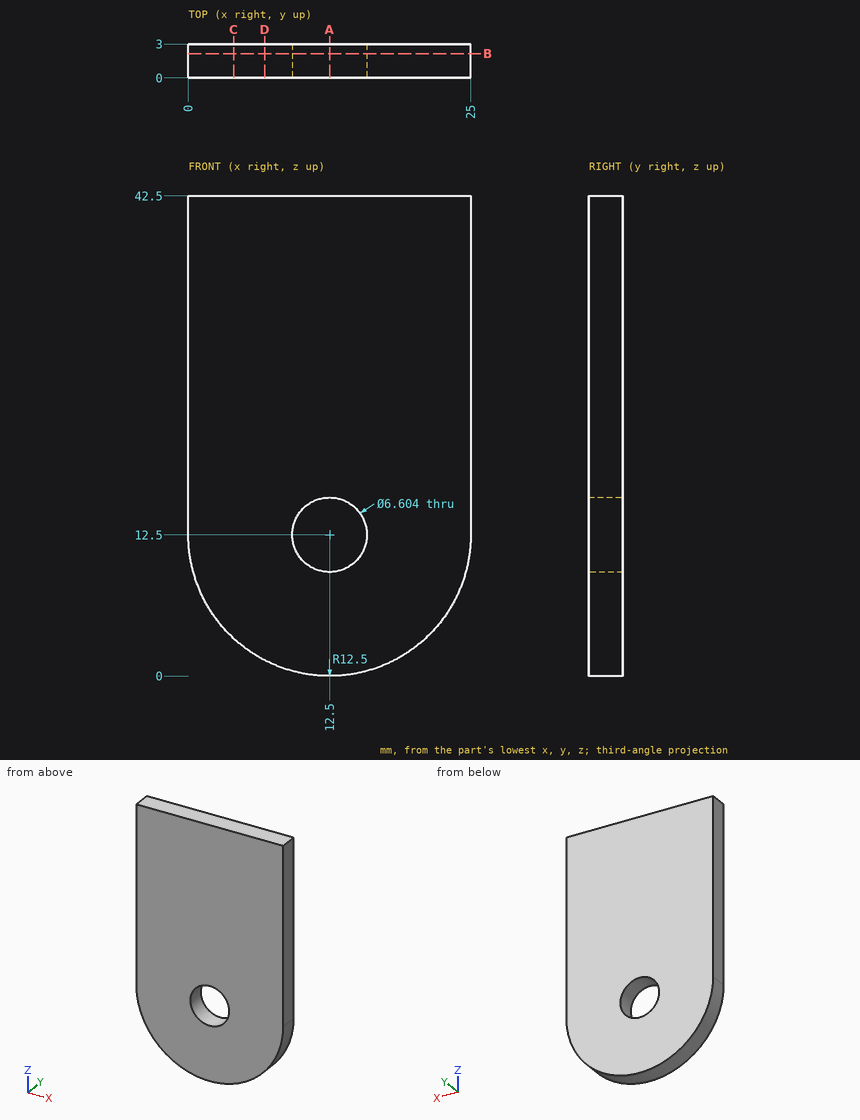
Job drawing, mm, ordinate dimensions from the low corner. One solid piece. Coordinates: 2 decimals unless noted, no trailing zeros. Write each loop counter-clockwise with the first axis right and the second up, starting at its lowest first coordinate (ties: lowest second). Pieces come first, ordered by that corner, then holes.
Item 1: Slice it at C-C (x = 4). Write the cut outline in (y, z), and give its area (3 significant figures).
Item 2: Slice it at B-B (y = 2.15). Write the cut outline in (x, z).
Item 3: Slice it at A-A (x = 12.5). Write the cut outline in (y, z).
Item 4: Probe line 1 (X direction, y = 2.25, z = 5); line 2 (Z direction, x = 16.5, y = 2.15); line 3 (X direction, y = 2.9, z = 9.5). List the from-to ranges inside material, lowest first.
Item 5: Pin check, flat tips, straight feed: pin 1 (1.5 mm diameter, centred on x = 4, y = 2.5, fed in from -Z); pin 2 (1 mm diameter, centred on y = 2, z = 4.5, fed in from +X). Stop position of each tip, or through.
Item 6: Slice it at D-D (x = 6.75). Write the cut outline in (y, z).
Results found:
1. outline: (0, 3.33) - (3, 3.33) - (3, 42.5) - (0, 42.5) - close
1. area: 117 mm2
2. outline: (0, 12.5) arc R12.5 ccw to (25, 12.5) - (25, 42.5) - (0, 42.5) - close; hole circle Ø6.6 at (12.5, 12.5)
3. outline: (0, 0) - (3, 0) - (3, 9.2) - (0, 9.2) - close; (0, 15.8) - (3, 15.8) - (3, 42.5) - (0, 42.5) - close
4. line 1: x = 2.5 to 22.5
4. line 2: z = 0.66 to 42.5
4. line 3: x = 0.37 to 11.12, 13.88 to 24.63
5. pin 1: stops at z = 2.69
5. pin 2: stops at x = 22.5
6. outline: (0, 1.4) - (3, 1.4) - (3, 42.5) - (0, 42.5) - close
